from build123d import *

# Parameters (mm, degrees)
F0_W          = 6
F0_H          = 120
F1_DEPTH      = 12.8
F1_DEPTH_BACK = 0.8
F2_R          = 2
F3_R          = 1
F4_R          = 1.15
F5_DEPTH      = 15
F6_W          = 3.8
F6_H          = 51
F6_R          = 2
F7_DEPTH      = 19
F8_R          = 3
F9_T1_DEPTH   = 13.6


# Not quite as in the source:
# - a fillet or chamfer that OpenCascade refuses, or shapes differently, is made with other operations: its cross-section is extruded or revolved along the edge and cut away or added


with BuildPart() as f1:
    # F0 (on Top) → F1 (new body, two sides)
    with BuildSketch(Plane.XY) as f1_sk:
        Polygon((2.9121718865, 60.9107007086), (-0.0878281135, 60.9107007086), (-0.0878281135, -59.0892992914), (2.9121718865, -59.0892992914), (2.9121718865, -56.0892992914), align=None)
        with Locations((-3.0878281135, 0.9107007086)):
            Rectangle(F0_W, F0_H)
        with BuildLine():
            Line((13.1121718865, -56.0892992914), (2.9121718865, -56.0892992914))
            Line((2.9121718865, -56.0892992914), (2.9121718865, -59.0892992914))
            Line((2.9121718865, -59.0892992914), (14.9121718865, -59.0892992914))
            ThreePointArc((14.9121718865, -59.0892992914), (25.3098855946, -51.9202262022), (37.9121718865, -51.0892992914))
            Line((37.9121718865, -51.0892992914), (37.9121718865, -48.0892992914))
            ThreePointArc((37.9121718865, -48.0892992914), (24.4865924683, -48.9100030948), (13.1121718865, -56.0892992914))
        make_face()
    extrude(amount=-F1_DEPTH)
    extrude(f1_sk.sketch, amount=F1_DEPTH_BACK)

    # F2
    f2_edges = [f1.edges().sort_by_distance(p)[0] for p in [
        (14.912172, -59.089299, -6),
    ]]
    fillet(f2_edges, radius=F2_R)

    # F3
    f3_edges = [f1.edges().sort_by_distance(p)[0] for p in [
        (2.912172, -56.089299, -6),
        (13.112172, -56.089299, -6),
        (37.912172, -48.089299, -6),
        (37.912172, -51.089299, -6),
    ]]
    fillet(f3_edges, radius=F3_R)

    # F4 (on face) → F5 (cut)
    with BuildSketch(Plane.YZ.offset(2.9121718865)):
        with Locations((-25.0892992914, -2)):
            Circle(F4_R)
        with Locations((-25.0892992914, -10)):
            Circle(F4_R)
        with Locations((45.8816848695, -2)):
            Circle(F4_R)
        with Locations((45.8816848695, -10)):
            Circle(F4_R)
    extrude(amount=-F5_DEPTH, mode=Mode.SUBTRACT)

    # F6 (on face) → F7 (cut)
    with BuildSketch(Plane.XY.offset(0.8)):
        with Locations((-1.25, 11.9107007086)):
            Rectangle(F6_W, F6_H)
        with Locations((-1, 54.3107017875)):
            Circle(F6_R)
    extrude(amount=-F7_DEPTH, mode=Mode.SUBTRACT)

    # F8
    f8_edges = [f1.edges().sort_by_distance(p)[0] for p in [
        (-6.087828, 60.910701, -6),
        (2.912172, 60.910701, -6),
        (-6.087828, -59.089299, -6),
    ]]
    fillet(f8_edges, radius=F8_R)

    # F9: fillet of radius 2 on 4 edges, made by hand

    # F9_s2 → F9_t1 (join)
    with BuildSketch(Plane.XY.offset(-12.8)):
        with BuildLine():
            ThreePointArc((-1.15, 37.4107007086), (-2.5642135624, 36.824914271), (-3.15, 35.4107007086))
            Line((-3.15, 35.4107007086), (-3.15, 37.4107007086))
            Line((-3.15, 37.4107007086), (-1.15, 37.4107007086))
        make_face()
        with BuildLine():
            ThreePointArc((0.65, 35.4107007086), (0.0642135624, 36.824914271), (-1.35, 37.4107007086))
            Line((-1.35, 37.4107007086), (0.65, 37.4107007086))
            Line((0.65, 37.4107007086), (0.65, 35.4107007086))
        make_face()
        with BuildLine():
            ThreePointArc((-3.15, -11.5892992914), (-2.5642135624, -13.0035128537), (-1.15, -13.5892992914))
            Line((-1.15, -13.5892992914), (-3.15, -13.5892992914))
            Line((-3.15, -13.5892992914), (-3.15, -11.5892992914))
        make_face()
        with BuildLine():
            ThreePointArc((0.65, -11.5892992914), (0.0642135624, -13.0035128537), (-1.35, -13.5892992914))
            Line((-1.35, -13.5892992914), (0.65, -13.5892992914))
            Line((0.65, -13.5892992914), (0.65, -11.5892992914))
        make_face()
    extrude(amount=F9_T1_DEPTH)


solid = f1.part
Check sheet for the modelled part. Datum: model origin and axes. Units: mm. A direction names the side the tool comes from. Round coordinates to 2 decimals unless told otherwise and drop trailing zeros. Order: outer loops, then holes, each group sorted by start corner. A loop starts at its lowest first (then second) coordinate and runs counter-clockwise, first axis right, second up.
Q1. Cross-section at B-B, the plane z = -10. Give the number of separate pieces and of enclosed holes in the cut face, plus the area to 3 significant figures.
Filled sheet:
separate pieces: 3
enclosed holes: 2
area: 945 mm2
Q2. Cross-section at A-A, the plane y = 32. Enter the section's corners in (x, z), plus the area to 3 significant figures.
Filled sheet:
outline: (-6.09, -12.8) - (-3.15, -12.8) - (-3.15, 0.8) - (-6.09, 0.8) - close; (0.65, -12.8) - (2.91, -12.8) - (2.91, 0.8) - (0.65, 0.8) - close
area: 70.7 mm2
Q3. Cross-section at C-C, the plane y = -15. Enter the section's corners in (x, z), plus the area to 3 significant figures.
Filled sheet:
outline: (-6.09, -12.8) - (2.91, -12.8) - (2.91, 0.8) - (-6.09, 0.8) - close
area: 122 mm2
Q4. Scan lines: L1, parallel to X at y = 17.5, z = -6.5; L2, parallel to X at y = 52, z = -8.25; L3, parallel to Y at x = 4, z = 0. Record each from-to range of solid material in increasing order.
Filled sheet:
L1: x = -6.09 to -3.15, 0.65 to 2.91
L2: x = -6.09 to 2.91
L3: y = -59.09 to -56.09
Q5. Draft check along Z on faces 4 (the face through (1, -12, -12.8)), 5 (the face through (-1.52, -26.24, -1.95)), 6 (the face through (25.014, -52.025, -6.095)), 7 (the face through (-1.5, -26, -10.7)). Enter one of: pulls with the +Z half, pulls with the -Z half, needs draft (parallel to the pull), parting line crosses it, or undercut.
Filled sheet:
face 4: pulls with the -Z half
face 5: undercut
face 6: needs draft
face 7: undercut
Q6. Cross-section at D-D, the plane x = 8.5. Enter the section's corners in (y, z), plus the area to 3 significant figures.
Filled sheet:
outline: (-59.09, -12.8) - (-56.09, -12.8) - (-56.09, 0.8) - (-59.09, 0.8) - close
area: 40.8 mm2
Q7. Set-up check for faces 1 (the face through (2.01, 60.055, -6.095)), 2 (the face through (8, -56.089, -6)), 3 (the face through (0.114, -12.952, -6.095)): record each of +Z, -Z, +X, -X, +Y, -Y from which the full face is reachable in a straight line by a thin tool's end or side.
Filled sheet:
face 1: +Z, -Z, +X, +Y
face 2: +Z, -Z, +Y
face 3: +Z, -Z
Q8. Depth check by flat-ended pin: P1, Ø3, axis at x = 33, z = -5, coming from the -Y side; P2, Ø4, axis at x = 26.5, z = -6.5, coming from the -Y side; P3, Ø4, axis at y = -14.5, z = -5.5, coming from the +X side; P4, Ø6, axis at x = 6, y = -1.5, coming from the -Z side. Enter the tip coordinate at first touch or a pass-through.
Filled sheet:
P1: stops at y = -50.66
P2: stops at y = -52.22
P3: stops at x = 2.91
P4: passes through
